```python
from build123d import *

# Parameters (mm, degrees)
F1_DEPTH  = 20
F2_R      = 47.5
F3_DEPTH  = 3
F4_R      = 35.5
F5_DEPTH  = 8
F6_R      = 35.5
F7_DEPTH  = 7
F7_TAPER  = 23
F8_R      = 32.5
F9_DEPTH  = 26
F10_R     = 14
F11_DEPTH = 8
F12_R     = 11.5
F13_DEPTH = 5
F15_DEPTH = 13
F16_R     = 2
F17_DEPTH = 70.001


with BuildPart() as f1:
    # F0 (on Front) → F1 (new body)
    with BuildSketch(Plane.XZ):
        with BuildLine():
            ThreePointArc((-17.5, 31.2409987036), (-18.0496972232, 28.9617871744), (-19.5779220779, 27.1837261447))
            ThreePointArc((-19.5779220779, 27.1837261447), (0, -33.5), (19.5779220779, 27.1837261447))
            ThreePointArc((19.5779220779, 27.1837261447), (18.0496972232, 28.9617871744), (17.5, 31.2409987036))
            Line((17.5, 31.2409987036), (17.5, 43.5657137142))
            Line((17.5, 43.5657137142), (0, 43.5657137142))
            Line((0, 43.5657137142), (-17.5, 43.5657137142))
            Line((-17.5, 43.5657137142), (-17.5, 31.2409987036))
        make_face()
    extrude(amount=-F1_DEPTH)

    # F2 (on face) → F3 (join)
    with BuildSketch(Plane.XZ):
        Circle(F2_R)
    extrude(amount=F3_DEPTH)

    # F4 (on face) → F5 (join)
    with BuildSketch(Plane.XZ.offset(3)):
        Circle(F4_R)
    extrude(amount=F5_DEPTH)

    # F6 (on face) → F7 (join)
    with BuildSketch(Plane.XZ.offset(11)):
        Circle(F6_R)
    extrude(amount=F7_DEPTH, taper=F7_TAPER)

    # F8 (on face) → F9 (join)
    with BuildSketch(Plane.XZ.offset(18)):
        Circle(F8_R)
    extrude(amount=F9_DEPTH)

    # F10 (on face) → F11 (join)
    with BuildSketch(Plane.XZ.offset(44)):
        Circle(F10_R)
    extrude(amount=F11_DEPTH)

    # F12 (on face) → F13 (join)
    with BuildSketch(Plane.XZ.offset(52)):
        Circle(F12_R)
    extrude(amount=F13_DEPTH)

    # F14 (on face) → F15 (join)
    with BuildSketch(Plane.XZ.offset(57)):
        Polygon((4.5744852646, 1.9992902459), (0.5558064898, 4.9612655713), (-4.0186787748, 2.9619753254), (-4.5744852646, -1.9992902459), (-0.5558064898, -4.9612655713), (4.0186787748, -2.9619753254), align=None)
    extrude(amount=F15_DEPTH)

    # F16 (on face) → F17 (cut, through all)
    with BuildSketch(Plane(origin=(0, 0, 0), x_dir=(-1, 0, 0), z_dir=(0, 1, 0))):
        with Locations((0, -40.5)):
            Circle(F16_R)
        with Locations((-35.0740288533, 20.25)):
            Circle(F16_R)
        with Locations((35.0740288533, 20.25)):
            Circle(F16_R)
    extrude(amount=-F17_DEPTH, mode=Mode.SUBTRACT)


solid = f1.part
```
Model file for the job. Use its own axes, mm. A direction names the side the tool comes from. Give positions to 0.01 mm unless a question says otherwise; leave off trailing zeros. Write each loop counter-clockwise with the first axis right and the second up, starting at its lowest first coordinate (ties: lowest second). Pieces come first, ordered by that corner, then holes. Notation, with made-up numbers: (69, 17) - (82, 17) arc R31 cw to (82, 45) - close; hole circle Ø2 at (75, -14.5). An arc over 180 degrees is marked (long way). One line per question, with ' | ' between items. Start each with the question number.
(1) Wall check: line 1 along X through (y, z) = (-1, 20); line 2 along Z through (x, y) = (0, -1.75); line 3 along Y through (x, z) = (-19, 4). Give the ranges that are in metal, low to high. Write a range as from..to.
(2) Two-plate mould, pull along Z, no slides. Class faces 5 (the face through (-1.5, -54.5, 11.4)), 6 (the face through (0, 10, 43.566)), 7 (the face through (33.166, -1.479, 20.851)): +Z half, -Z half, draft (parallel to the pull), parting line (faces both ways), or undercut.
(3) Slice it at D-D on y = -54.5. Write the cut outline in (x, z), plus the area to 3 significant figures.
(4) Slice it at B-B on y = -28. Write the cut outline in (x, z).
(5) Pin check, flat tips, straight feed: P1, Ø4.5, axis at x = -35.07, z = 20.25, coming from the -Y side; P2, Ø6, axis at y = 8, z = 39, coming from the +X side; P3, Ø5, axis at y = -22.5, z = -16.5, coming from the +X side; P4, Ø11.5, axis at x = 3.5, z = 3, coming from the -Y side. Stop position of each tip, or through.
(6) Slice it at C-C on z = 20.25. Give the number of separate pieces and of enclosed holes in the cut face, plus the area to 3 significant figures.
(7) 3-axis set-ups, long thin cutter, end or side, ignore diameter. For faces 1 (the face through (2.59, -63.41, 3.46)), 2 (the face through (-18.035, 9.86, 28.991)), 3 (the face through (2, -52, 11.5)), 4 (the face through (-4.293, -63.409, 0.516)): which of +Z, -Z, +X, -X, +Y, -Y reach the whole face in a straight line?
(8) Slice it at A-A on z = -40.5. Write the cut outline in (x, y).
Results below:
1) line 1: -43.08..-37.06, -33.09..33.09, 37.06..43.08 | line 2: -47.5..-42.5, -38.5..47.5 | line 3: -44..20
2) face 5: parting line | face 6: +Z half | face 7: undercut
3) outline: circle Ø23 at (0, 0) | area: 415 mm^2
4) outline: circle Ø65 at (0, 0)
5) P1: y = -3 | P2: x = 17.5 | P3: x = 29.33 | P4: y = -70
6) separate pieces: 3 | enclosed holes: 0 | area: 3,470 mm^2
7) face 1: +Z, +X, -Y | face 2: +Z, -X, +Y | face 3: -Y | face 4: +Z, -X, -Y
8) outline: (-24.82, -3) - (-2, -3) - (-2, 0) - (-24.82, 0) - close; (2, -3) - (24.82, -3) - (24.82, 0) - (2, 0) - close
